The listing builds one solid part. Answer for the finished solid, in the listing's coordinates (mm). A direction names the side the tool comes from. Coordinates: 2 decimals unless noted, no trailing zeros. Loops run counter-clockwise (first coordinate to the right, second up) from the corner with the lowest first, then second, coordinate; pieces in that order, holes last. Notation, with made-up numbers: (-5, -23) - (20, -23) arc R17 ccw to (20, -6) - close; hole circle Ø3 at (-25.5, 35). An arc over 180 degrees is marked (long way). Return JSON: item names as keys, results as strings. Group by question number.
1. Find the intervals of material crossed by line 1 along Z through (x, y) = (711, 22.25); line 2 along Z through (x, y) = (454, 2); line 3 along X through (y, z) = (8.25, 59.5), in increasing order.
2. Section B-B (x = 670) is taken. Write down the section's boundary in (y, z), and give its area (3 significant figures).
3. Each of these flat-tipped pins is pushed along its axis until it touches: P1, Ø8, axis at x = 711.02, z = -92.65, coming from the +Y side; P2, Ø3, axis at x = 171, y = 3.5, coming from the -Z side; P3, Ø13, axis at x = 711.02, z = -92.65, coming from the -Y side; P4, Ø9, axis at x = 709.5, z = -451, coming from the +Y side. Where does it stop, or does it pass through?
4. Section C-C (z = 146.5) is taken. Write down the section's boundary in (x, y), and give its area (3 significant figures).
5. Section A-A (y = 6.25) is taken. State how many separate pieces and enclosed holes the cut face has, and give its area (3 significant figures).
6. The mould has two halves that part along Z. Classify faces 4 (the face through (435.503, 12.878, -426.913)), 5 (the face through (-256, 13, -346.655)), 6 (the face through (169, 25.4, -129)): pulls with the +Z half, pulls with the -Z half, needs draft (parallel to the pull), parting line crosses it, or undercut.
7. Which of the six approach directions +Z, -Z, +X, -X, +Y, -Y give full straight-line access (tool end or side, diameter ignored) to faces 1 (the face through (169, 0, -129)), 2 (the face through (481.663, 12.878, -333.069)), 3 (the face through (-101.78, 13, -394))?
```python
from build123d import *

# Parameters (mm, degrees)
SKETCH2_W                                     = 2006.6
SKETCH2_H                                     = 762
BOSS_EXTRUDE1_DEPTH                           = 25.4
CUT_EXTRUDE18_DEPTH                           = 26.4
F_1_4_20_TAPPED_HOLE1_D                       = 5.1054
SKETCH4_R                                     = 215.9
CUT_EXTRUDE1_DEPTH                            = 26.4
SKETCH26_W                                    = 381
SKETCH26_H                                    = 82.55
CUT_EXTRUDE2_DEPTH                            = 26.4
SKETCH109_R                                   = 50.8
CUT_EXTRUDE15_DEPTH                           = 26.4
SKETCH48_W                                    = 304.8
SKETCH48_H                                    = 95.25
CUT_EXTRUDE9_DEPTH                            = 26.4
CUT_EXTRUDE12_DEPTH                           = 26.4
CUT_EXTRUDE13_DEPTH                           = 26.4
CUT_EXTRUDE17_DEPTH                           = 26.4
CBORE_FOR_1_4_SOCKET_HEAD_CAP_SCREW1_AT_COUNT = 2
CBORE_FOR_1_4_SOCKET_HEAD_CAP_SCREW1_AT_PITCH = 558.8
CBORE_FOR_1_4_SOCKET_HEAD_CAP_SCREW1_2_COUNT  = 2
CBORE_FOR_1_4_SOCKET_HEAD_CAP_SCREW1_2_PITCH  = 366.324009587
CBORE_FOR_1_4_SOCKET_HEAD_CAP_SCREW1_3_COUNT  = 2
CBORE_FOR_1_4_SOCKET_HEAD_CAP_SCREW1_3_PITCH  = 274.74300719
CBORE_FOR_1_4_SOCKET_HEAD_CAP_SCREW1_4_COUNT  = 2
CBORE_FOR_1_4_SOCKET_HEAD_CAP_SCREW1_4_PITCH  = 840.889624148
CBORE_FOR_1_4_SOCKET_HEAD_CAP_SCREW1_5_COUNT  = 2
CBORE_FOR_1_4_SOCKET_HEAD_CAP_SCREW1_5_PITCH  = 762


with BuildPart() as part:
    # Sketch2 → Boss-Extrude1 (new body)
    with BuildSketch(Plane(origin=(0, 0, 0), x_dir=(1, 0, 0), z_dir=(0, 1, 0))):
        with Locations((596.720248579, 143.454782609)):
            Rectangle(SKETCH2_W, SKETCH2_H)
    extrude(amount=BOSS_EXTRUDE1_DEPTH)

    # Sketch120 → Cut-Extrude18 (cut, through all)
    with BuildSketch(Plane(origin=(0, 25.4, 0), x_dir=(1, 0, 0), z_dir=(0, 1, 0))):
        with BuildLine():
            Line((364.731895319, 486.354782609), (761.820248579, 486.354782609))
            Line((761.820248579, 486.354782609), (761.820248579, 524.454782609))
            Line((761.820248579, 524.454782609), (368.120248579, 524.454782609))
            ThreePointArc((368.120248579, 524.454782609), (367.271491927, 505.329596742), (364.731895319, 486.354782609))
        make_face()
    extrude(amount=-CUT_EXTRUDE18_DEPTH, mode=Mode.SUBTRACT)

    # 1/4-20 Tapped Hole1 (through all)
    with Locations(Plane(origin=(0, 25.4, 0), x_dir=(1, 0, 0), z_dir=(0, 1, 0))):
        with Locations((736.420248579, 473.948827926)):
            Hole(F_1_4_20_TAPPED_HOLE1_D / 2)

    # Sketch4 → Cut-Extrude1 (cut, through all)
    with BuildSketch(Plane(origin=(0, 25.4, 0), x_dir=(1, 0, 0), z_dir=(0, 1, 0))):
        with Locations((152.220248579, 524.454782609)):
            Circle(SKETCH4_R)
    extrude(amount=-CUT_EXTRUDE1_DEPTH, mode=Mode.SUBTRACT)

    # Sketch26 → Cut-Extrude2 (cut, through all)
    with BuildSketch(Plane(origin=(0, 25.4, 0), x_dir=(1, 0, 0), z_dir=(0, 1, 0))):
        with Locations((-216.079751421, 483.179782609)):
            Rectangle(SKETCH26_W, SKETCH26_H)
    extrude(amount=-CUT_EXTRUDE2_DEPTH, mode=Mode.SUBTRACT)

    # Sketch109 → Cut-Extrude15 (cut, through all)
    with BuildSketch(Plane(origin=(0, 25.4, 0), x_dir=(1, 0, 0), z_dir=(0, 1, 0))):
        with Locations((469.720248579, 194.254782609)):
            Circle(SKETCH109_R)
    extrude(amount=-CUT_EXTRUDE15_DEPTH, mode=Mode.SUBTRACT)

    # Sketch48 → Cut-Extrude9 (cut, through all)
    with BuildSketch(Plane(origin=(0, 25.4, 0), x_dir=(1, 0, 0), z_dir=(0, 1, 0))):
        with Locations((-254.179751421, 394.279782609)):
            Rectangle(SKETCH48_W, SKETCH48_H)
    extrude(amount=-CUT_EXTRUDE9_DEPTH, mode=Mode.SUBTRACT)

    # Sketch56 → Cut-Extrude12 (cut, through all)
    with BuildSketch(Plane(origin=(0, 25.4, 0), x_dir=(1, 0, 0), z_dir=(0, 1, 0))):
        with BuildLine():
            Line((512.462825882, 400.413315761), (152.220248579, 524.454782609))
            Line((152.220248579, 524.454782609), (439.764598644, 274.496292563))
            ThreePointArc((439.764598644, 274.496292563), (482.175927421, 333.954782609), (512.462825882, 400.413315761))
        make_face()
    extrude(amount=-CUT_EXTRUDE12_DEPTH, mode=Mode.SUBTRACT)

    # Sketch105 → Cut-Extrude13 (cut, through all)
    with BuildSketch(Plane(origin=(0, 25.4, 0), x_dir=(1, 0, 0), z_dir=(0, 1, 0))):
        with BuildLine():
            Line((152.220248579, -237.545217391), (-406.579751421, -237.545217391))
            Line((-406.579751421, -237.545217391), (-406.579751421, 6.394400028))
            ThreePointArc((-406.579751421, 6.394400028), (-152.64200595, -173.902579895), (152.220248579, -237.545217391))
        make_face()
    extrude(amount=-CUT_EXTRUDE13_DEPTH, mode=Mode.SUBTRACT)

    # Sketch111 → Cut-Extrude17 (cut, through all)
    with BuildSketch(Plane(origin=(0, 25.4, 0), x_dir=(1, 0, 0), z_dir=(0, 1, 0))):
        with BuildLine():
            Line((761.820248579, 67.254782609), (761.820248579, 524.454782609))
            Line((761.820248579, 524.454782609), (1600.020248579, 524.454782609))
            Line((1600.020248579, 524.454782609), (1600.020248579, -237.545217391))
            Line((1600.020248579, -237.545217391), (152.220248579, -237.545217391))
            ThreePointArc((152.220248579, -237.545217391), (492.99700835, -157.098736933), (761.820248579, 67.254782609))
        make_face()
    extrude(amount=-CUT_EXTRUDE17_DEPTH, mode=Mode.SUBTRACT)

    # Sketch123 → CBORE for 1/4 Socket Head Cap Screw1 (revolve, cut)
    with BuildSketch(Plane(origin=(-50.979751421, 25.4, -92.654782609), x_dir=(0, 0, 1), z_dir=(1, 0, 0))):
        Polygon((0, 0), (0, 25.4), (3.3782, 25.4), (3.3782, 6.35), (5.55625, 6.35), (5.55625, 2.2225), (7.77875, 0), align=None)
    cbore_for_1_4_socket_head_cap_screw1 = revolve(axis=Axis((-50.979751421, 31.75, -92.654782609), (0, -1, 0)), mode=Mode.SUBTRACT)

    # CBORE for 1/4 Socket Head Cap Screw1 at: CBORE for 1/4 Socket Head Cap Screw1 ×2
    with Locations(*[(i * CBORE_FOR_1_4_SOCKET_HEAD_CAP_SCREW1_AT_PITCH, 0, 0) for i in range(1, CBORE_FOR_1_4_SOCKET_HEAD_CAP_SCREW1_AT_COUNT)]):
        add(cbore_for_1_4_socket_head_cap_screw1, mode=Mode.SUBTRACT)

    # CBORE for 1_4 Socket Head Cap Screw1 2: CBORE for 1/4 Socket Head Cap Screw1 ×2
    with Locations(*[Vector(-0.832050294, 0, -0.554700196) * (i * CBORE_FOR_1_4_SOCKET_HEAD_CAP_SCREW1_2_PITCH) for i in range(1, CBORE_FOR_1_4_SOCKET_HEAD_CAP_SCREW1_2_COUNT)]):
        add(cbore_for_1_4_socket_head_cap_screw1, mode=Mode.SUBTRACT)

    # CBORE for 1_4 Socket Head Cap Screw1 3: CBORE for 1/4 Socket Head Cap Screw1 ×2
    with Locations(*[Vector(-0.832050294, 0, 0.554700196) * (i * CBORE_FOR_1_4_SOCKET_HEAD_CAP_SCREW1_3_PITCH) for i in range(1, CBORE_FOR_1_4_SOCKET_HEAD_CAP_SCREW1_3_COUNT)]):
        add(cbore_for_1_4_socket_head_cap_screw1, mode=Mode.SUBTRACT)

    # CBORE for 1_4 Socket Head Cap Screw1 4: CBORE for 1/4 Socket Head Cap Screw1 ×2
    with Locations(*[Vector(0.90618314, 0, -0.422885465) * (i * CBORE_FOR_1_4_SOCKET_HEAD_CAP_SCREW1_4_PITCH) for i in range(1, CBORE_FOR_1_4_SOCKET_HEAD_CAP_SCREW1_4_COUNT)]):
        add(cbore_for_1_4_socket_head_cap_screw1, mode=Mode.SUBTRACT)

    # CBORE for 1_4 Socket Head Cap Screw1 5: CBORE for 1/4 Socket Head Cap Screw1 ×2
    with Locations(*[(i * CBORE_FOR_1_4_SOCKET_HEAD_CAP_SCREW1_5_PITCH, 0, 0) for i in range(1, CBORE_FOR_1_4_SOCKET_HEAD_CAP_SCREW1_5_COUNT)]):
        add(cbore_for_1_4_socket_head_cap_screw1, mode=Mode.SUBTRACT)


solid = part.part
```
The answers:
{
 "1": {"line 1": "z = -486.35 to -453.81, -442.7 to -98.21, -87.1 to -6.37", "line 2": "z = -486.35 to -420.54, -291.88 to -242.56, -145.95 to 175.24", "line 3": "x = -337.31 to -282.95, -276.21 to 641.75"},
 "2": {"outline": "(0, -486.35) - (25.4, -486.35) - (25.4, 34.61) - (0, 34.61) - close", "area": "13,200 mm2"},
 "3": {"P1": "stops at y = 19.05", "P2": "stops at z = -309.51", "P3": "stops at y = 0", "P4": "stops at y = 25.26"},
 "4": {"outline": "(-208.98, 0) - (513.42, 0) - (513.42, 25.4) - (-208.98, 25.4) - close", "area": "18,300 mm2"},
 "5": {"separate pieces": "1", "enclosed holes": "8", "area": "619,000 mm2"},
 "6": {"face 4": "undercut", "face 5": "pulls with the -Z half", "face 6": "needs draft"},
 "7": {"face 1": "+Z, -Z, +X, -X, -Y", "face 2": "+Y, -Y", "face 3": "-Z, -X, +Y, -Y"}
}
